Check sheet for the modelled part. Datum: model origin and axes. Units: mm. A direction names the side the tool comes from. Round coordinates to 2 decimals unless told otherwise and drop trailing zeros. Order: outer loops, then holes, each group sorted by start corner. A loop starts at its lowest first (then second) coordinate and runs counter-clockwise, first axis right, second up. Notation, with made-up numbers: (-22.75, 20.5) -> (8.25, 20.5) arc R14 ccw to (8.25, 37.5) -> close; hole circle Ø9 at (0, 31.25). An arc over 180 degrees is marked (long way). Use CSV: the item, a comma, the result in double quotes.
```python
from build123d import *

# Parameters (mm, degrees)
F0_W     = 30
F0_H     = 10
F1_DEPTH = 40
F2_W     = 30
F2_H     = 10
F3_DEPTH = 20
F4_W     = 24
F4_H     = 10
F5_DEPTH = 6


with BuildPart() as f1:
    # F0 (on Top) → F1 (new body)
    with BuildSketch(Plane.XY):
        Rectangle(F0_W, F0_H)
    extrude(amount=F1_DEPTH)

    # F2 (on face) → F3 (join)
    with BuildSketch(Plane.XY.offset(40)):
        Rectangle(F2_W, F2_H)
    extrude(amount=F3_DEPTH)

    # F4 (on face) → F5 (join)
    with BuildSketch(Plane.XY.offset(60)):
        Rectangle(F4_W, F4_H)
    extrude(amount=F5_DEPTH)


solid = f1.part
```
Q1. Mould release check, pull along Z, two halves, no side actions. Record for faces 1 (the face through (13, 0, 60)), 2 (the face through (0, 0, 0)), 3 (the face through (-12, 0, 63)): pulls with the +Z half, pulls with the -Z half, needs draft (parallel to the pull), parting line crosses it, or undercut.
Result sheet:
face 1,"pulls with the +Z half"
face 2,"pulls with the -Z half"
face 3,"needs draft"
Q2. Go/stop test with flat-tipped pins: pin 1 (0.9 mm diameter, centred on x = -13.5, y = -2, fed in from +Z); pin 2 (3 mm diameter, centred on y = -1.5, z = 63, fed in from -X). Record where each tip stops, or that it passes through.
Result sheet:
pin 1,"stops at z = 60"
pin 2,"stops at x = -12"
Q3. Access from +Z, -Z, +X, -X, +Y, -Y to the whole of each face (thin tool, end or side, straight path). Record for faces 4 (the face through (-14, 0, 60)), 5 (the face through (12, 0, 63)), 6 (the face through (0, -5, 33)).
Result sheet:
face 4,"+Z, -X, +Y, -Y"
face 5,"+Z, +X, +Y, -Y"
face 6,"+Z, -Z, +X, -X, -Y"
Q4. Sectioned sample at A-A, the plane y = -1.25. Enter the section's corners in (x, z).
Result sheet:
outline,"(-15, 0) -> (15, 0) -> (15, 60) -> (12, 60) -> (12, 66) -> (-12, 66) -> (-12, 60) -> (-15, 60) -> close"
Q5. Scan lines: L1, parallel to X at y = 3.75, z = 63; L2, parallel to Z at x = 13.25, y = 3.5. Record each from-to range of solid material in increasing order.
Result sheet:
L1,"x = -12 to 12"
L2,"z = 0 to 60"
